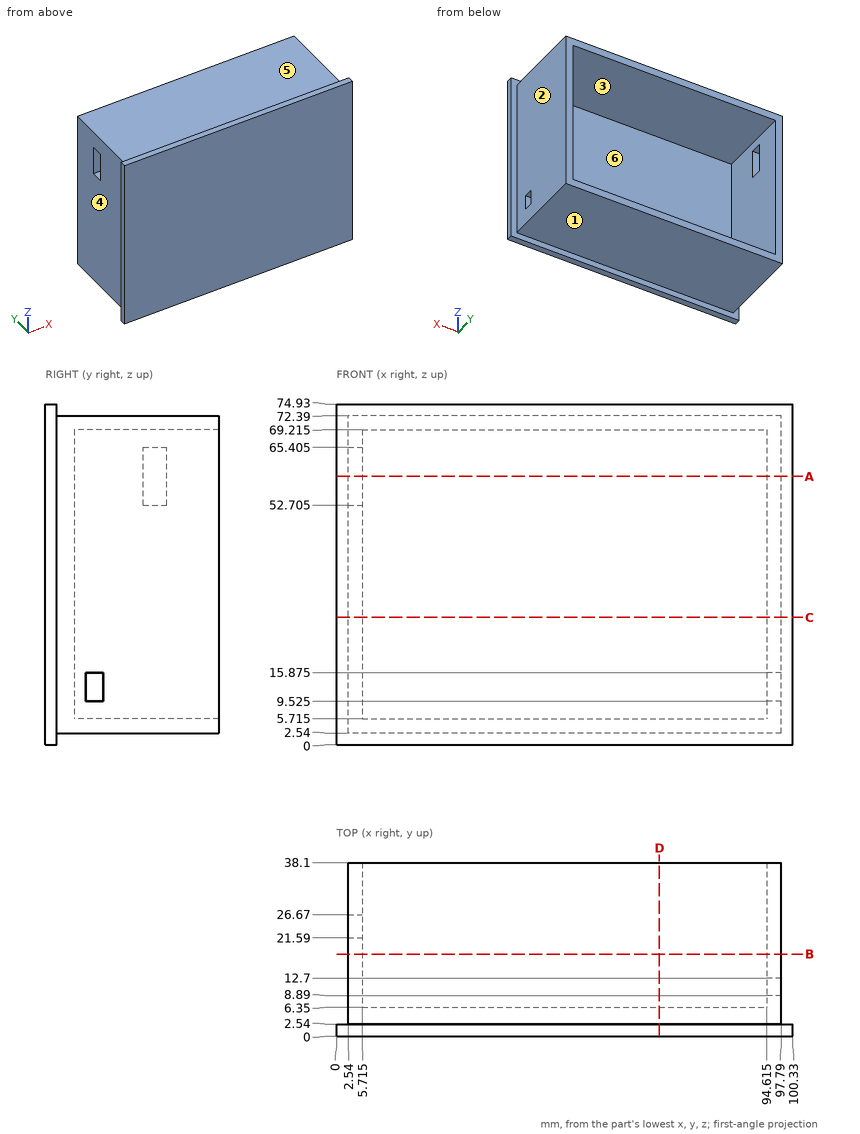
Can you work these out from the drawing? Everything is in mm from the part's minimum corner. A direction names the side the tool comes from. Give positions to 0.01 mm unless a question says otherwise; leave off trailing zeros. Order: outer loops, then holes, each group sorted by start corner. A loop starts at its lowest first (then second) coordinate and runs counter-clockwise, first axis right, second up. Notation, with made-up numbers: M 40,71 L 74,71 A9 ccw 74,84 Z; hole C 73,-18 d1. An arc over 180 degrees is marked long. Use a Markdown table: item, result. Add a question column.
Item 1: Suppose I cut it at C-C (z = 28). List the corners of the cut face in (x, y) for me (3 decimals), then the cut area to 3 significant figures.
Item 2: Will these pins go through, and if not, where does the flat tip stop? pin 1 (10.5 mm diameter, centred on y = 13.5, z = 33.5, fed in from -X); pin 2 (1 mm diameter, centred on x = 50, z = 36, fed in from -Y); pin 3 (3 mm diameter, centred on x = 82.5, z = 52.5, fed in from +Y); pin 4 (1.6 mm diameter, centred on x = 96, y = 10, fed in from -Z).
Item 3: We'd pull the mould along Z, two halves only. Please class the marked faces 4, 5 and 6: +Z half, -Z half, draft (parallel to the pull), parting line (faces both ways), or undercut.
Item 4: Suppose I cut it at A-A (z = 59). List the corners of the cut face in (x, y) for me (3 decimals).
Item 5: For the marked faces 1, 2 and 3, which set-ups out of +Z, -Z, +X, -X, +Y, -Y let a thin tool reach every point of the face, with its end or its side?
Item 6: Suppose I cut it at B-B (y = 18). List the corners of the cut face in (x, z) for me (3 decimals).
Item 7: Suppose I cut it at D-D (x = 71). List the corners of the cut face in (y, z) for me (3 decimals).
Item 8: If I drill on L1, parallel to X at y = 21, z = 58.5 (3 decimals); L2, parallel to Z at x = 14.5, y = 30 (3 decimals); L3, parallel to X at y = 3, z = 10.5, over which ranges is the centre line in solid material (lowest first)? Write a range as [from, to].
Answer sheet:
| question | item | result |
|---|---|---|
| 1 | outline | M 0,0 L 100.33,0 L 100.33,2.54 L 97.79,2.54 L 97.79,38.1 L 94.615,38.1 L 94.615,6.35 L 5.715,6.35 L 5.715,38.1 L 2.54,38.1 L 2.54,2.54 L 0,2.54 Z |
| 1 | area | 819 mm² |
| 2 | pin 1 | stops at x = 2.54 |
| 2 | pin 2 | stops at y = 0 |
| 2 | pin 3 | stops at y = 6.35 |
| 2 | pin 4 | stops at z = 2.54 |
| 3 | face 4 | draft |
| 3 | face 5 | +Z half |
| 3 | face 6 | undercut |
| 4 | outline | M 0,0 L 100.33,0 L 100.33,2.54 L 97.79,2.54 L 97.79,38.1 L 94.615,38.1 L 94.615,6.35 L 5.715,6.35 L 5.715,21.59 L 2.54,21.59 L 2.54,2.54 L 0,2.54 Z; M 2.54,26.67 L 5.715,26.67 L 5.715,38.1 L 2.54,38.1 Z |
| 5 | face 1 | -Z, +X, -X, +Y |
| 5 | face 2 | +Z, -Z, +X, +Y |
| 5 | face 3 | +Y |
| 6 | outline | M 2.54,2.54 L 97.79,2.54 L 97.79,72.39 L 2.54,72.39 Z; hole M 5.715,5.715 L 94.615,5.715 L 94.615,69.215 L 5.715,69.215 Z |
| 7 | outline | M 0,0 L 2.54,0 L 2.54,2.54 L 38.1,2.54 L 38.1,5.715 L 6.35,5.715 L 6.35,69.215 L 38.1,69.215 L 38.1,72.39 L 2.54,72.39 L 2.54,74.93 L 0,74.93 Z |
| 8 | L1 | x = [2.54, 5.715], [94.615, 97.79] |
| 8 | L2 | z = [2.54, 5.715], [69.215, 72.39] |
| 8 | L3 | x = [2.54, 97.79] |
